Geometry: final body of the model. Coordinates: model frame, mm. Give positions to 0.01 mm unless a question says otherwise; leave off trailing zeros. Loops run counter-clockwise (first coordinate to the right, second up) from the corner with the lowest first, then second, coordinate; pieces in that order, holes last.
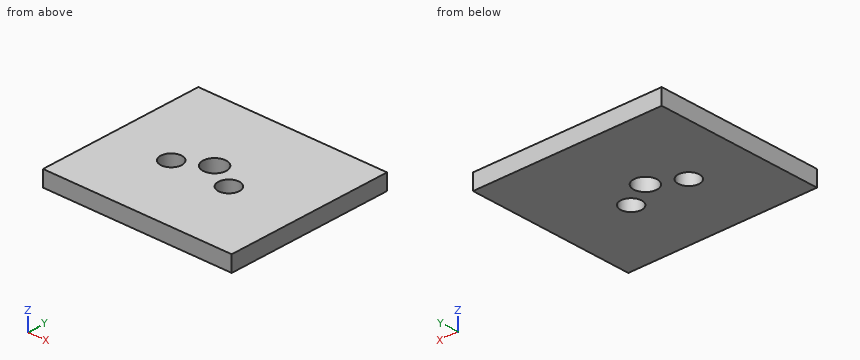
from build123d import *

# Parameters (mm, degrees)
CYLINDER008_R     = 2.2
CYLINDER008_DEPTH = 10
CYLINDER007_R     = 2
CYLINDER007_DEPTH = 10
CYLINDER006_R     = 2
CYLINDER006_DEPTH = 10
BOX004_W          = 36
BOX004_H          = 32
BOX004_DEPTH      = 3


with BuildPart() as cylinder008:
    # Cylinder008 → Cylinder008 (new body)
    with BuildSketch(Plane(origin=(17, 17, 0), x_dir=(1, 0, 0), z_dir=(0, 0, 1))):
        Circle(CYLINDER008_R)
    extrude(amount=CYLINDER008_DEPTH)


with BuildPart() as cylinder007:
    # Cylinder007 → Cylinder007 (new body)
    with BuildSketch(Plane(origin=(22.5, 14, 0), x_dir=(1, 0, 0), z_dir=(0, 0, 1))):
        Circle(CYLINDER007_R)
    extrude(amount=CYLINDER007_DEPTH)


with BuildPart() as cylinder006:
    # Cylinder006 → Cylinder006 (new body)
    with BuildSketch(Plane(origin=(11.5, 14, 0), x_dir=(1, 0, 0), z_dir=(0, 0, 1))):
        Circle(CYLINDER006_R)
    extrude(amount=CYLINDER006_DEPTH)


with BuildPart() as manual_valve_plate:
    # Box004 → Box004 (new body)
    with BuildSketch(Plane.XY):
        with Locations((18, 16)):
            Rectangle(BOX004_W, BOX004_H)
    extrude(amount=BOX004_DEPTH)

    # Cut: cut Cylinder006
    add(cylinder006.part, mode=Mode.SUBTRACT)

    # Cut007: cut Cylinder007
    add(cylinder007.part, mode=Mode.SUBTRACT)

    # Cut008: cut Cylinder008
    add(cylinder008.part, mode=Mode.SUBTRACT)


solid = manual_valve_plate.part
Item 1: Ray query, probe 1 along X at (y, z) = (14, 0.9); probe 2 along Y at (x, z) = (11.5, 1); probe 3 along X at (y, z) = (17, 0.9). Return the intervals inside material, ascending.
Values follow:
probe 1: x = 0 to 9.5, 13.5 to 20.5, 24.5 to 36
probe 2: y = 0 to 12, 16 to 32
probe 3: x = 0 to 14.8, 19.2 to 36
Item 2: Section query A-A on y = 14. Return loops of the section in (x, z).
Values follow:
outline: (0, 0) - (9.5, 0) - (9.5, 3) - (0, 3) - close; (13.5, 0) - (20.5, 0) - (20.5, 3) - (13.5, 3) - close; (24.5, 0) - (36, 0) - (36, 3) - (24.5, 3) - close
Item 3: Pin query (flat end, axial travel): pin 1 (1 mm diameter, centred on y = 26.5, z = 1.5, fed in from -X). Return the tip coordinate at first contact, or that it passes through.
Values follow:
pin 1: stops at x = 0
Item 4: Section query C-C on z = 1.85. Return loops of the section in (x, y).
Values follow:
outline: (0, 0) - (36, 0) - (36, 32) - (0, 32) - close; hole circle Ø4 at (11.5, 14); hole circle Ø4.4 at (17, 17); hole circle Ø4 at (22.5, 14)
Item 5: Section query D-D on x = 22.5. Return loops of the section in (y, z).
Values follow:
outline: (0, 0) - (12, 0) - (12, 3) - (0, 3) - close; (16, 0) - (32, 0) - (32, 3) - (16, 3) - close
Item 6: Section query B-B on x = 17. Return loops of the section in (y, z).
Values follow:
outline: (0, 0) - (14.8, 0) - (14.8, 3) - (0, 3) - close; (19.2, 0) - (32, 0) - (32, 3) - (19.2, 3) - close
